Build history of the part. All positions in model axes, mm. Round coordinates to 2 decimals unless told otherwise and drop trailing zeros. Loops run counter-clockwise (first coordinate to the right, second up) from the corner with the lowest first, then second, coordinate; pieces in that order, holes last. Notation, with made-up numbers: (62, -20) - (110, -20) arc R23 ccw to (110, -8) - close; hole circle Ø6 at (25.5, 88). An arc over 180 degrees is marked (long way). Use a Markdown table: item, result.
from build123d import *

# Parameters (mm, degrees)
F1_DEPTH = 38.1


with BuildPart() as f1:
    # F0 (on Front) → F1 (new body)
    with BuildSketch(Plane.XZ):
        with BuildLine():
            Line((-63.295935, 13.055353), (-63.295935, -5.994647))
            Line((-63.295935, -5.994647), (63.704065, -5.994647))
            Line((63.704065, -5.994647), (63.704065, 13.055353))
            ThreePointArc((63.704065, 13.055353), (52.526578, 19.557037), (40.691665, 24.766922))
            Line((40.691665, 24.766922), (40.691665, 16.714011))
            ThreePointArc((40.691665, 16.714011), (38.304065, 8.686553), (35.916465, 16.714011))
            Line((35.916465, 16.714011), (35.916465, 26.438266))
            ThreePointArc((35.916465, 26.438266), (0.204065, 32.105353), (-35.508335, 26.438266))
            Line((-35.508335, 26.438266), (-35.508335, 23.897591))
            Line((-35.508335, 23.897591), (-35.508335, 16.561381))
            ThreePointArc((-35.508335, 16.561381), (-37.895935, 8.813553), (-40.283535, 16.561381))
            Line((-40.283535, 16.561381), (-40.283535, 24.766922))
            ThreePointArc((-40.283535, 24.766922), (-52.118449, 19.557037), (-63.295935, 13.055353))
        make_face()
    extrude(amount=F1_DEPTH)


solid = f1.part
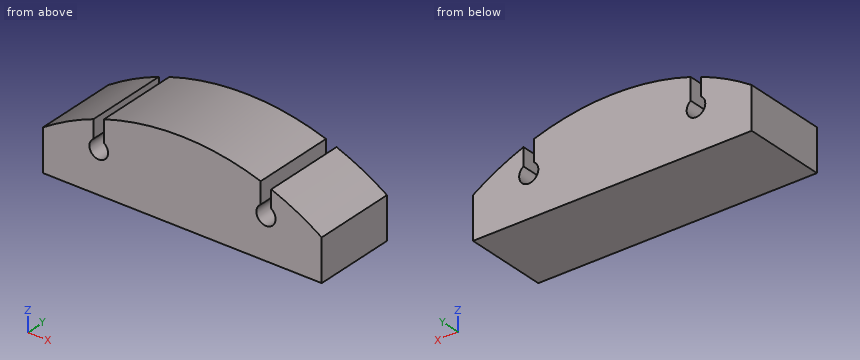
Q1. Drop flat-ended pins along their axis: pin 1 (1.5 mm diameter, centred on x = 7, y = -10.5, fed in from +Z); pin 2 (6.5 mm diameter, centred on y = -20, z = 20.5, fed in from +X); pin 3 (10.5 mm diameter, centred on y = -21, z = 21, fed in from +X). Give the stop position or say it passes through.
Results found:
| item | result |
|---|---|
| pin 1 | stops at z = 31.95 |
| pin 2 | stops at x = 56.83 |
| pin 3 | stops at x = 59.42 |
Q2. Cut at B-B, the plane y = -27.5. List the corners of the cut face in (x, z), plus the area to 3 significant figures.
Results found:
| item | result |
|---|---|
| outline | (-63.3, -5.99) - (63.7, -5.99) - (63.7, 13.06) arc R115.36 ccw to (40.69, 24.77) - (40.69, 16.71) arc R4.37 cw (long way) to (35.92, 16.71) - (35.92, 26.44) arc R115.36 ccw to (-35.51, 26.44) - (-35.51, 16.56) arc R4.24 cw (long way) to (-40.28, 16.56) - (-40.28, 24.77) arc R115.36 ccw to (-63.3, 13.06) - close |
| area | 3,860 mm2 |
Q3. Cut at C-C, the plane z = 10. List the corners of the cut face in (x, y), plus the area to 3 significant figures.
Results found:
| item | result |
|---|---|
| outline | (-63.3, -38.1) - (-40.84, -38.1) - (-40.84, 0) - (-63.3, 0) - close; (-34.95, -38.1) - (35.18, -38.1) - (35.18, 0) - (-34.95, 0) - close; (41.43, -38.1) - (63.7, -38.1) - (63.7, 0) - (41.43, 0) - close |
| area | 4,380 mm2 |
Q4. Cut at D-D, the plane x = 53. List the corners of the cut face in (y, z).
Results found:
| item | result |
|---|---|
| outline | (-38.1, -5.99) - (0, -5.99) - (0, 19.31) - (-38.1, 19.31) - close |
Q5. Cut at A-A, the plane z = 23. List the corners of the cut face in (x, y), plus the area to 3 significant figures.
Results found:
| item | result |
|---|---|
| outline | (-44.72, -38.1) - (-40.28, -38.1) - (-40.28, 0) - (-44.72, 0) - close; (-35.51, -38.1) - (35.92, -38.1) - (35.92, 0) - (-35.51, 0) - close; (40.69, -38.1) - (45.12, -38.1) - (45.12, 0) - (40.69, 0) - close |
| area | 3,060 mm2 |
Q6. Probe line 1 (X direction, y = -33, z = 22); line 2 (X direction, y = -2.5, z = 23.5); line 3 (Z direction, x = -1, y = -33). List the from-to ranges inside material, lowest first.
Results found:
| item | result |
|---|---|
| line 1 | x = -47.01 to -40.28, -35.51 to 35.92, 40.69 to 47.42 |
| line 2 | x = -43.51 to -40.28, -35.51 to 35.92, 40.69 to 43.92 |
| line 3 | z = -5.99 to 32.1 |
